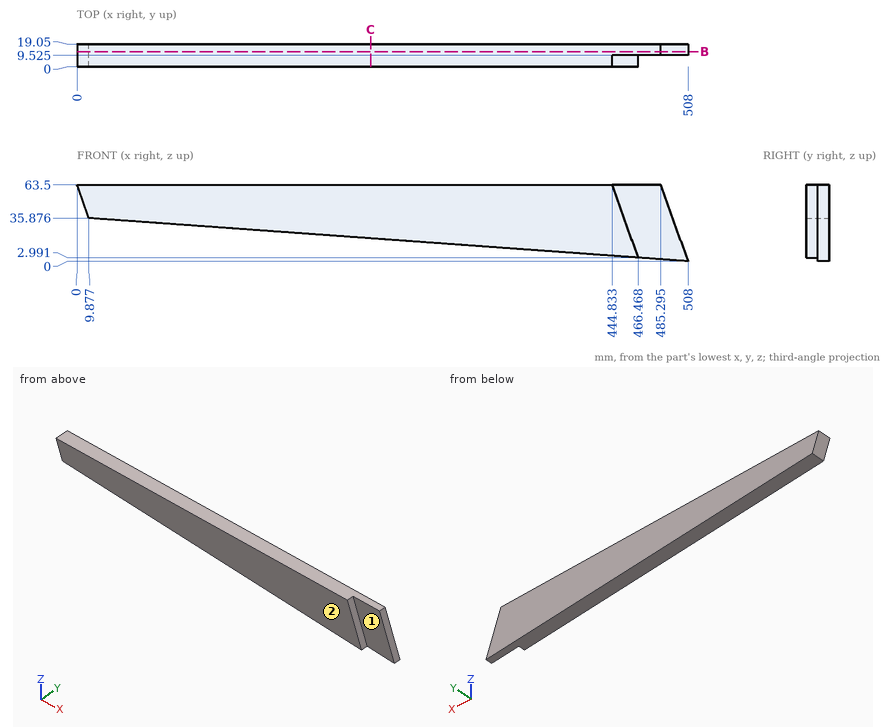
Could you check a few things on this drawing? It's one solid part, dimensions in mm from its lowest x, y, z. A direction names the side the tool comes from. Coordinates: 2 decimals unless noted, no trailing zeros. Order: outer loops, then holes, each group sorted by start corner. A loop starts at its lowest first (then second) coordinate and runs counter-clockwise, first axis right, second up.
1. If we section it at B-B (y = 12.75): Please give me the cut outline in (x, z) (1 decimal), then the cut area to 3 significant figures.
2. I'm going to push flat-ended pins straight in: pin 1 (6 mm diameter, centred on x = 130.5, y = 7.5, fed in from -Z); pin 2 (6 mm diameter, centred on x = 103, y = 16, fed in from -Z). Where does each tip first touch, or does it pass through?
3. If we section it at C-C (x = 244): Please give me the cut outline in (y, z).
4. I need wall thicknesses on line 1 (Z direction, x = 259, y = 8.5); line 2 (Z direction, x = 63.5, y = 10.5); line 3 (X direction, y = 15.75, z = 49.5) (1 decimal). Which ranges of each line are inside material? Lowest first, please.
5. For the marked faces 1 and 2, which set-ups out of +Z, -Z, +X, -X, +Y, -Y let a thin tool reach every point of the face, with its end or its side?
Entries:
1. outline: (0, 63.5) - (9.9, 35.9) - (508, 0) - (485.3, 63.5) - close
1. area: 22,100 mm2
2. pin 1: stops at z = 26.97
2. pin 2: stops at z = 28.95
3. outline: (0, 19.01) - (19.05, 19.01) - (19.05, 63.5) - (0, 63.5) - close
4. line 1: z = 17.93 to 63.5
4. line 2: z = 32.01 to 63.5
4. line 3: x = 5 to 490.3
5. face 1: +Z, +X, -Y
5. face 2: +Z, -Z, +X, -X, -Y
